```python
from build123d import *

# Parameters (mm, degrees)
SKETCH003_W     = 40
SKETCH003_H     = 40
PAD002_DEPTH    = 2.2
SKETCH004_W     = 2.5
SKETCH004_H     = 40
PAD003_DEPTH    = 30
SKETCH005_W     = 40
SKETCH005_H     = 2.2
PAD004_DEPTH    = 20
SKETCH006_R     = 1.5
POCKET001_DEPTH = 5
CHAMFER001_SIZE = 2
FILLET001_R     = 2
SKETCH007_R     = 1.5
POCKET002_DEPTH = 5


with BuildPart() as part:
    # Sketch003 → Pad002 (new body)
    with BuildSketch(Plane.XY):
        with Locations((-30, 30)):
            Rectangle(SKETCH003_W, SKETCH003_H)
    extrude(amount=PAD002_DEPTH)

    # Sketch004 (on Face6 of Pad002) → Pad003 (join)
    with BuildSketch(Plane.XY.offset(2.2)):
        with Locations((-48.75, 30)):
            Rectangle(SKETCH004_W, SKETCH004_H)
    extrude(amount=PAD003_DEPTH)

    # Sketch005 (on Face4 of Pad003) → Pad004 (join)
    with BuildSketch(Plane.YZ.offset(-47.5)):
        with Locations((30, 31.1)):
            Rectangle(SKETCH005_W, SKETCH005_H)
    extrude(amount=PAD004_DEPTH)

    # Sketch006 (on Face10 of Pad004) → Pocket001 (cut)
    with BuildSketch(Plane.XY.offset(32.2)):
        with Locations((-40, 40)):
            Circle(SKETCH006_R)
        with Locations((-40, 20)):
            Circle(SKETCH006_R)
    extrude(amount=-POCKET001_DEPTH, mode=Mode.SUBTRACT)

    # Chamfer001
    chamfer001_edges = [part.edges().sort_by_distance(p)[0] for p in [
        (-47.5, 30, 2.2),
        (-47.5, 30, 30),
    ]]
    chamfer(chamfer001_edges, length=CHAMFER001_SIZE)

    # Fillet001
    fillet001_edges = [part.edges().sort_by_distance(p)[0] for p in [
        (-27.5, 10, 31.1),
        (-10, 10, 1.1),
        (-27.5, 50, 31.1),
        (-10, 50, 1.1),
    ]]
    fillet(fillet001_edges, radius=FILLET001_R)

    # Sketch007 (on Face5 of Fillet001) → Pocket002 (cut)
    with BuildSketch(Plane(origin=(0, 0, 0), x_dir=(1, 0, 0), z_dir=(0, 0, -1))):
        with Locations((-43, -15.8)):
            Circle(SKETCH007_R)
        with Locations((-14.7, -15.8)):
            Circle(SKETCH007_R)
        with Locations((-43, -44.2)):
            Circle(SKETCH007_R)
        with Locations((-14.7, -44.2)):
            Circle(SKETCH007_R)
    extrude(amount=-POCKET002_DEPTH, mode=Mode.SUBTRACT)


solid = part.part
```
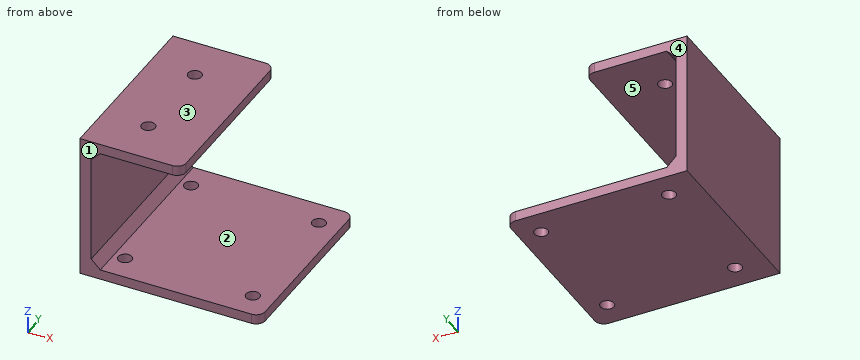
Check sheet for the modelled part. Datum: model origin and axes. Units: mm. Face numbers are marked on the shaded views. A direction names the side the tool comes from. Round coordinates to 2 decimals unless told otherwise and drop trailing zeros. Order: outer loops, then holes, each group sorted by start corner. A loop starts at its lowest first (then second) coordinate and runs counter-clockwise, first axis right, second up. Notation, with made-up numbers: (28.25, 11.25) -> (39.25, 11.25) arc R24 ccw to (39.25, 38.25) -> close; hole circle Ø6 at (-3.5, 46). An arc over 180 degrees is marked (long way). Use CSV: the item, a comma, the result in double quotes.
(1) Draft check along Z on the marked faces 1, 2 and 3. Enter one of: pulls with the +Z half, pulls with the -Z half, needs draft (parallel to the pull), parting line crosses it, or undercut.
Worked out:
face 1,"needs draft"
face 2,"undercut"
face 3,"pulls with the +Z half"
(2) Material ranges on line 1 along Y through (x, z) = (-43, 1.15); line 2 along Y through (x, z) = (-40, 31); line 3 along Z through (x, y) = (-45.5, 20), recorded low to high. Write a range as from..to.
Worked out:
line 1,"10..14.3, 17.3..42.7, 45.7..50"
line 2,"10..18.5, 21.5..38.5, 41.5..50"
line 3,"0..2.2, 30..32.2"
(3) Depth check by flat-ended pin: pin 1 (6 mm diameter, centred on x = -18.5, y = 44, fed in from +Z); pin 2 (19 mm diameter, centred on y = 20, z = 22, fed in from +X); pin 3 (1.8 mm diameter, centred on x = -43, y = 15.8, fed in from -Z). Enter the tip coordinate at first touch or a pass-through.
Worked out:
pin 1,"z = 2.2"
pin 2,"x = -27.5"
pin 3,"z = 30"
(4) Tool access check on the marked faces 4 and 5. Record the directions out of +Z, -Z, +X, -X, +Y, -Y that give a thin tool (end or side, any length) a straight path to the whole face; none if there is none.
Worked out:
face 4,"+Z, -Z, +X, -X, +Y"
face 5,"+X, +Y, -Y"
(5) Cross-section at D-D (x = -40). Record the boundary of the cut face in (y, z).
Worked out:
outline,"(10, 0) -> (50, 0) -> (50, 2.2) -> (10, 2.2) -> close; (10, 30) -> (18.5, 30) -> (18.5, 32.2) -> (10, 32.2) -> close; (21.5, 30) -> (38.5, 30) -> (38.5, 32.2) -> (21.5, 32.2) -> close; (41.5, 30) -> (50, 30) -> (50, 32.2) -> (41.5, 32.2) -> close"
(6) Cross-section at C-C (y = 34.5). Record the boundary of the cut face in (x, z).
Worked out:
outline,"(-50, 0) -> (-10, 0) -> (-10, 2.2) -> (-45.5, 2.2) -> (-47.5, 4.2) -> (-47.5, 28) -> (-45.5, 30) -> (-27.5, 30) -> (-27.5, 32.2) -> (-50, 32.2) -> close"
(7) Cross-section at B-B (x = -14.7). Record the boundary of the cut face in (y, z).
Worked out:
outline,"(10, 0) -> (14.3, 0) -> (14.3, 2.2) -> (10, 2.2) -> close; (17.3, 0) -> (42.7, 0) -> (42.7, 2.2) -> (17.3, 2.2) -> close; (45.7, 0) -> (50, 0) -> (50, 2.2) -> (45.7, 2.2) -> close"
(8) Cross-section at A-A (x = -31.5). Record the boundary of the cut face in (y, z).
Worked out:
outline,"(10, 0) -> (50, 0) -> (50, 2.2) -> (10, 2.2) -> close; (10, 30) -> (50, 30) -> (50, 32.2) -> (10, 32.2) -> close"
